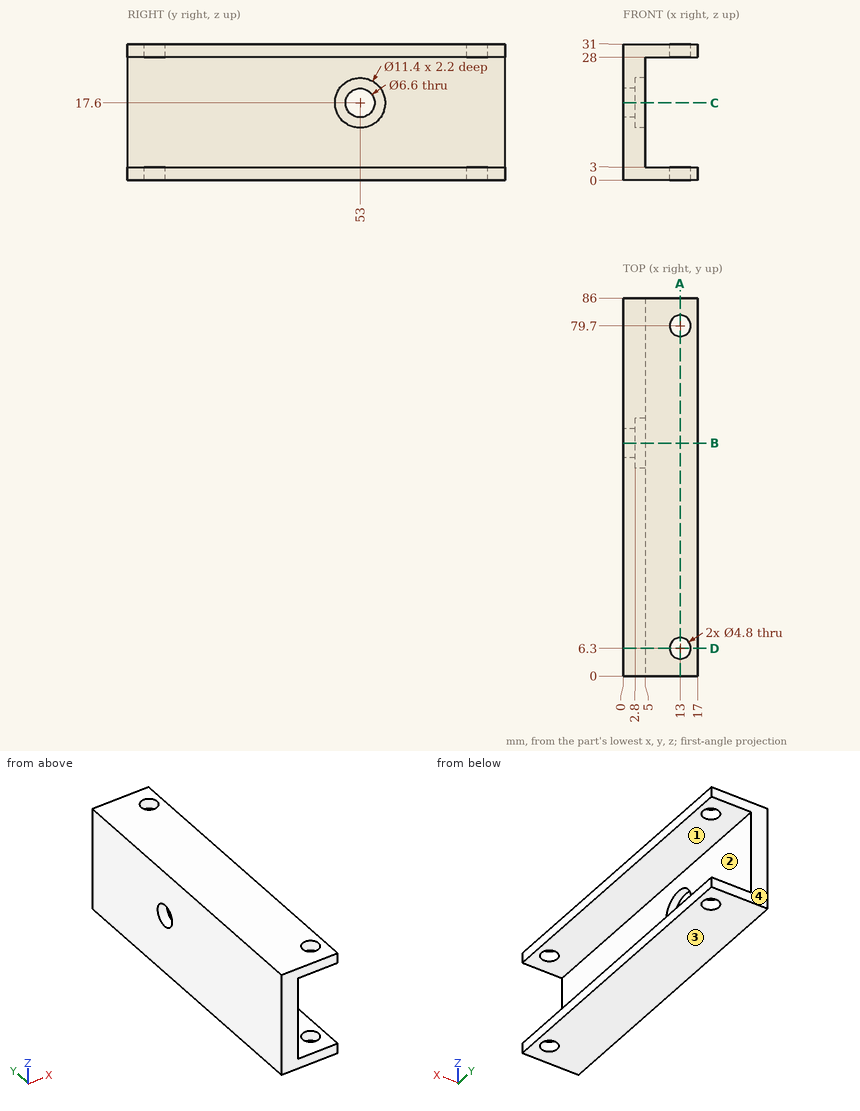
Source: three-view drawing plus pictorial views. Frame: mm from the lowest corner of the part. Round coordinates to 2 decimals unless told otherwise and drop trailing zeros. Loops run counter-clockwise (first coordinate to the right, second up) from the corner with the lowest first, then second, coordinate; pieces in that order, holes last. Notation, with made-up numbers: (31, -19.75) -> (69, -19.75) arc R24 cw to (69, -9.75) -> close; hole circle Ø1 at (81, 12.25). An arc over 180 degrees is marked (long way). Use one line per item in the form item = value.
Item 1: Cut plane B-B on y = 53. Output: boundary loops of the cut face in (x, z), then the cut area to 3 significant figures.
Evaluation:
outline = (0, 0) -> (17, 0) -> (17, 3) -> (5, 3) -> (5, 11.9) -> (2.8, 11.9) -> (2.8, 14.3) -> (0, 14.3) -> close; (0, 20.9) -> (2.8, 20.9) -> (2.8, 23.3) -> (5, 23.3) -> (5, 28) -> (17, 28) -> (17, 31) -> (0, 31) -> close
area = 183 mm2
Item 2: Material intervals for probe 1 along Y at (x, z) = (13, 30.2); probe 2 along Z at (x, y) = (11.5, 56.5); probe 3 along X at (y, z) = (6, 29), sorted ascending.
Evaluation:
probe_1 = 0 to 3.9, 8.7 to 77.3, 82.1 to 86
probe_2 = 0 to 3, 28 to 31
probe_3 = 0 to 10.62, 15.38 to 17
Item 3: Cut plane D-D on y = 6.3. Output: boundary loops of the cut face in (x, z).
Evaluation:
outline = (0, 0) -> (10.6, 0) -> (10.6, 3) -> (5, 3) -> (5, 28) -> (10.6, 28) -> (10.6, 31) -> (0, 31) -> close; (15.4, 0) -> (17, 0) -> (17, 3) -> (15.4, 3) -> close; (15.4, 28) -> (17, 28) -> (17, 31) -> (15.4, 31) -> close
Item 4: Cut plane C-C on z = 17.6. Output: boundary loops of the cut face in (x, y), then the cut area to 3 significant figures.
Evaluation:
outline = (0, 0) -> (5, 0) -> (5, 47.3) -> (2.8, 47.3) -> (2.8, 49.7) -> (0, 49.7) -> close; (0, 56.3) -> (2.8, 56.3) -> (2.8, 58.7) -> (5, 58.7) -> (5, 86) -> (0, 86) -> close
area = 386 mm2
Item 5: Cut plane A-A on x = 13. Output: boundary loops of the cut face in (y, z).
Evaluation:
outline = (0, 0) -> (3.9, 0) -> (3.9, 3) -> (0, 3) -> close; (0, 28) -> (3.9, 28) -> (3.9, 31) -> (0, 31) -> close; (8.7, 0) -> (77.3, 0) -> (77.3, 3) -> (8.7, 3) -> close; (8.7, 28) -> (77.3, 28) -> (77.3, 31) -> (8.7, 31) -> close; (82.1, 0) -> (86, 0) -> (86, 3) -> (82.1, 3) -> close; (82.1, 28) -> (86, 28) -> (86, 31) -> (82.1, 31) -> close
Item 6: Contact query for flat-ended pins moving along their axis: pin 1 Ø4 at (x, y) = (13, 79.7) entering from +Z; pin 2 Ø7.5 at (y, z) = (33, 13.5) entering from +X; pin 3 Ø3.5 at (y, z) = (53.5, 20) entering from +X. Output: stop coordinate, or through.
Evaluation:
pin_1 = through
pin_2 = 5
pin_3 = 2.8
Item 7: Draft query along Z for the marked faces 1, 2, 3 and 4. Return one class per face: released by +Z, released by -Z, zero draft, split by the parting line, or undercut.
Evaluation:
face_1 = undercut
face_2 = undercut
face_3 = released by -Z
face_4 = zero draft
